Geometry: final body of the model. Coordinates: model frame, mm. A direction names the side the tool comes from. Give positions to 0.01 mm unless a question says otherwise; leave off trailing zeros. Write each loop counter-clockwise with the first axis right and the second up, starting at its lowest first coordinate (ties: lowest second). Pieces come first, ordered by that corner, then holes. Notation, with made-up numbers: M 46,35.5 L 78,35.5 A22 cw 78,55.5 Z; hole C -35.5,49.25 d9. An arc over 180 degrees is marked long. Use a Markdown table: item, result. Add a question column.
1) Section C-C on y = 13. Return the cut outline in (x, z).
2) Draft query along Y for faces 3 (the flat face through (-10.173, 11.368, -93.916)), 4 (the cylindrical face through (-4.15, 5.01, -93.92)), 5 (the flat face through (-6, 19.05, -94)). Return one class per face: +Y half, -Y half, draft (parallel to the pull), parting line (faces both ways), or undercut.
3) Section A-A on x = -9. Return the cut outline in (y, z), then the cut area to 3 significant figures.
4) Set-up query: faces 1 (the flat face through (-9.23, 12.23, -93.92)), 2 (the flat face through (-8.1, 11, 0)). Return all of +Z, -Z, +X, -X, +Y, -Y with unobstructed straight access to the full face (end or side cutting, diameter ignored); none if empty.
5) Pin query (flat end, axial travel): pin 1 (3 mm diameter, centred on y = 8, z = -26, fed in from +X); pin 2 (1.5 mm diameter, centred on y = 15.5, z = -102.5, fed in from -X); pin 3 (8 mm diameter, centred on y = 11.5, z = -130.5, fed in from -X). Return the tip coordinate at first contact, or that it passes through.
6) Line query: line 1 (Y direction, x = -0.75, z = -24.5); line 2 (Y direction, x = -10, z = -76.5); line 3 (X direction, y = 3.75, z = -161). Output: solid intervals per line, ascending.
7) Section D-D on y = 5. Return the cut outline in (x, z), then the cut area to 3 significant figures.
```python
from build123d import *

# Parameters (mm, degrees)
EXTRUDE_THIN1_DEPTH = 190.5
FILLET1_R           = 1.27


with BuildPart() as part:
    # Sketch2 → Extrude-Thin1 (new body)
    with BuildSketch(Plane.XY):
        with BuildLine():
            Line((0, 19.05), (-12.7, 19.05))
            ThreePointArc((-12.7, 19.05), (-14.933416251, 17.494706059), (-14.249357426, 14.860479244))
            Line((-14.249357426, 14.860479244), (-5.98022255, 7.775342526))
            ThreePointArc((-5.98022255, 7.775342526), (-3.936796637, 4.112343257), (-4.7625, 0))
            Line((-4.7625, 0), (0, 0))
            Line((0, 0), (0, 1.27))
            Line((0, 1.27), (-2.845784509, 1.27))
            ThreePointArc((-2.845784509, 1.27), (-2.920461936, 5.33839935), (-5.153898589, 8.739753596))
            Line((-5.153898589, 8.739753596), (-13.423033466, 15.824890314))
            ThreePointArc((-13.423033466, 15.824890314), (-13.742260917, 17.054196161), (-12.7, 17.78))
            Line((-12.7, 17.78), (0, 17.78))
            Line((0, 17.78), (0, 19.05))
        make_face()
    extrude(amount=-EXTRUDE_THIN1_DEPTH)

    # Fillet1
    fillet1_edges = [part.edges().sort_by_distance(p)[0] for p in [
        (-4.7625, 0, -95.25),
    ]]
    fillet(fillet1_edges, radius=FILLET1_R)


solid = part.part
```
Found:
| question | item | result |
|---|---|---|
| 1 | outline | M -12.08,-190.5 L -10.13,-190.5 L -10.13,0 L -12.08,0 Z |
| 2 | face 3 | -Y half |
| 2 | face 4 | undercut |
| 2 | face 5 | +Y half |
| 3 | outline | M 10.36,-190.5 L 12.04,-190.5 L 12.04,0 L 10.36,0 Z; M 17.78,-190.5 L 19.05,-190.5 L 19.05,0 L 17.78,0 Z |
| 3 | area | 561 mm² |
| 4 | face 1 | +Z, -Z, +X |
| 4 | face 2 | +Z, +X, -X, +Y, -Y |
| 5 | pin 1 | x = -3.39 |
| 5 | pin 2 | x = -15.04 |
| 5 | pin 3 | x = -14.77 |
| 6 | line 1 | 0 to 1.27, 17.78 to 19.05 |
| 6 | line 2 | 11.22 to 12.89, 17.78 to 19.05 |
| 6 | line 3 | -3.89 to -2.62 |
| 7 | outline | M -4.15,-190.5 L -2.82,-190.5 L -2.82,0 L -4.15,0 Z |
| 7 | area | 252 mm² |
